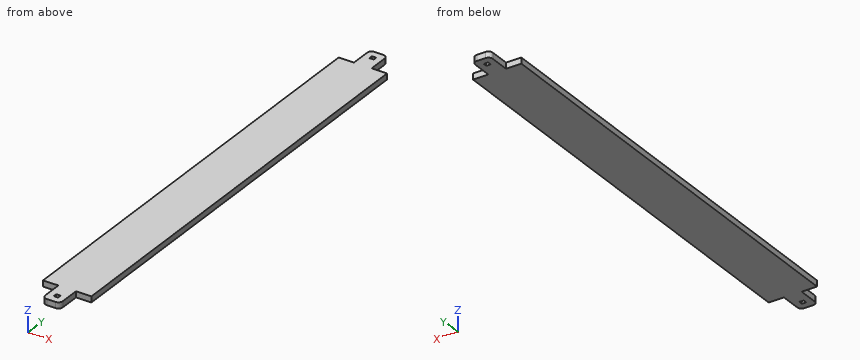
from build123d import *

# Parameters (mm, degrees)
F1_DEPTH = 27


with BuildPart() as f1:
    # F0 (on Top) → F1 (new body)
    with BuildSketch(Plane.XY):
        with BuildLine():
            Line((70, 1016), (0, 1016))
            Line((0, 1016), (0, 0))
            Line((0, 0), (220, 0))
            Line((220, 0), (220, 1016))
            Line((220, 1016), (150.000581, 1016.285126))
            Line((150.000581, 1016.285126), (150.000581, 1106.285126))
            ThreePointArc((150.000581, 1106.285126), (144.142716, 1120.427261), (130.000581, 1126.285126))
            Line((130.000581, 1126.285126), (90, 1126.285126))
            ThreePointArc((90, 1126.285126), (75.857864, 1120.427261), (70, 1106.285126))
            Line((70, 1106.285126), (70, 1016))
        make_face()
        with BuildLine():
            Line((120.00029, 1076.285126), (110.00029, 1076.285126))
            Line((110.00029, 1076.285126), (100.00029, 1076.285126))
            Line((100.00029, 1076.285126), (100.00029, 1091.285126))
            ThreePointArc((100.00029, 1091.285126), (110.00029, 1094.271711), (120.00029, 1091.285126))
            Line((120.00029, 1091.285126), (120.00029, 1076.285126))
        make_face(mode=Mode.SUBTRACT)
        with BuildLine():
            Line((220, 0), (0, 0))
            Line((0, 0), (0, -1016))
            Line((0, -1016), (70, -1016))
            Line((70, -1016), (70, -1106.285126))
            ThreePointArc((70, -1106.285126), (75.857864, -1120.427261), (90, -1126.285126))
            Line((90, -1126.285126), (130.000581, -1126.285126))
            ThreePointArc((130.000581, -1126.285126), (144.142716, -1120.427261), (150.000581, -1106.285126))
            Line((150.000581, -1106.285126), (150.000581, -1016.285126))
            Line((150.000581, -1016.285126), (220, -1016))
            Line((220, -1016), (220, 0))
        make_face()
        with BuildLine():
            Line((120.00029, -1076.285126), (120.00029, -1091.285126))
            ThreePointArc((120.00029, -1091.285126), (110.00029, -1094.271711), (100.00029, -1091.285126))
            Line((100.00029, -1091.285126), (100.00029, -1076.285126))
            Line((100.00029, -1076.285126), (110.00029, -1076.285126))
            Line((110.00029, -1076.285126), (120.00029, -1076.285126))
        make_face(mode=Mode.SUBTRACT)
    extrude(amount=F1_DEPTH)


solid = f1.part
CAD build for the part. Positions are in the model's coordinates, mm. Round coordinates to 2 decimals unless told otherwise and drop trailing zeros. Write each loop counter-clockwise with the first axis right and the second up, starting at its lowest first coordinate (ties: lowest second). Pieces come first, ordered by that corner, then holes. Notation, with made-up numbers: M -11,45 L 22,45 A14 ccw 22,50 Z; hole C 0.5,-39.75 d10. An arc over 180 degrees is marked long. Use a Markdown table: item, result. Add a question column.
1. Flat gauge pins, fed straight in: P1, Ø13.5, axis at y = -1042, z = 9, coming from the -X side; P2, Ø7.5, axis at y = -1084.5, z = 15, coming from the +X side; P3, Ø13.5, axis at x = 28.5, z = 11, coming from the -Y side. Where does each tip first touch, or does it go through?
2. Slice it at A-A on z = 9. Give the cut face in (x, y).
3. Slice it at B-B on x = 23. Give the cut face in (y, z).
4. Drill centre lines: probe 1 along Y at (x, z) = (203.5, 4); probe 2 along Y at (x, z) = (23, 16); probe 3 along X at (y, z) = (1022, 8.75). Where is each one in solid material? Low to high.
Reply:
| question | item | result |
|---|---|---|
| 1 | P1 | stops at x = 70 |
| 1 | P2 | stops at x = 150 |
| 1 | P3 | stops at y = -1016 |
| 2 | outline | M 0,-1016 L 70,-1016 L 70,-1106.29 A20 ccw 90,-1126.29 L 130,-1126.29 A20 ccw 150,-1106.29 L 150,-1016.29 L 220,-1016 L 220,1016 L 150,1016.29 L 150,1106.29 A20 ccw 130,1126.29 L 90,1126.29 A20 ccw 70,1106.29 L 70,1016 L 0,1016 Z; hole M 100,-1091.29 A18.23 ccw 120,-1091.29 L 120,-1076.29 L 100,-1076.29 Z; hole M 100,1076.29 L 120,1076.29 L 120,1091.29 A18.23 ccw 100,1091.29 Z |
| 3 | outline | M -1016,0 L 1016,0 L 1016,27 L -1016,27 Z |
| 4 | probe 1 | y = -1016.07 to 1016.07 |
| 4 | probe 2 | y = -1016 to 1016 |
| 4 | probe 3 | x = 70 to 150 |
